Read the model definition and answer for the solid it produces. Units are mm, in the model's axes. Face numbers are marked on the shaded views. A direction names the side the tool comes from. Coordinates: 2 decimals unless noted, no trailing zeros. Order: outer loops, then holes, each group sorted by start corner. A loop starts at its lowest first (then second) coordinate and runs counter-clockwise, first axis right, second up. Notation, with made-up numbers: M 16.25,31 L 67.25,31 A33 cw 67.25,65 Z; hole C -28,31.25 d10. An arc over 180 degrees is marked long. Put each result on its own line as item: value.
from build123d import *

# Parameters (mm, degrees)
SKETCH_1_R          = 3
EXTRUDE_1_DEPTH     = 17
SKETCH_2_R          = 1.5
EXTRUDE_2_DEPTH     = 5
CHAMFER_1_SIZE      = 0.5
SKETCH_3_R          = 1.5
SKETCH_3_R_2        = 1.25
CUT_EXTRUDE_3_DEPTH = 1.5
SKETCH_4_W          = 2
SKETCH_4_H          = 2
CUT_EXTRUDE_4_DEPTH = 10
CHAMFER_2_SIZE      = 0.5


with BuildPart() as part:
    # 草图1 → 拉伸1 (new body)
    with BuildSketch(Plane.XY):
        Circle(SKETCH_1_R)
    extrude(amount=EXTRUDE_1_DEPTH)

    # 草图2 → 拉伸2 (add)
    with BuildSketch(Plane.XY.offset(17)):
        Circle(SKETCH_2_R)
    extrude(amount=EXTRUDE_2_DEPTH)

    # 倒角1
    chamfer_1_edges = [part.edges().sort_by_distance(p)[0] for p in [
        (-1.5, 0, 22),
    ]]
    chamfer(chamfer_1_edges, length=CHAMFER_1_SIZE)

    # 草图3 → 拉伸3 (cut)
    with BuildSketch(Plane.XY.offset(17)):
        Circle(SKETCH_3_R)
        Circle(SKETCH_3_R_2, mode=Mode.SUBTRACT)
    extrude(amount=CUT_EXTRUDE_3_DEPTH, mode=Mode.SUBTRACT)

    # 草图4 → 拉伸4 (cut, symmetric)
    with BuildSketch(Plane(origin=(0, 0, 0), x_dir=(0, 0, -1), z_dir=(1, 0, 0))):
        with Locations((-1, 0)):
            Rectangle(SKETCH_4_W, SKETCH_4_H)
    extrude(amount=CUT_EXTRUDE_4_DEPTH, both=True, mode=Mode.SUBTRACT)

    # 倒角2
    chamfer_2_edges = [part.edges().sort_by_distance(p)[0] for p in [
        (0, 3, 0),
        (0, -3, 0),
        (-3, 0, 17),
    ]]
    chamfer(chamfer_2_edges, length=CHAMFER_2_SIZE)


solid = part.part
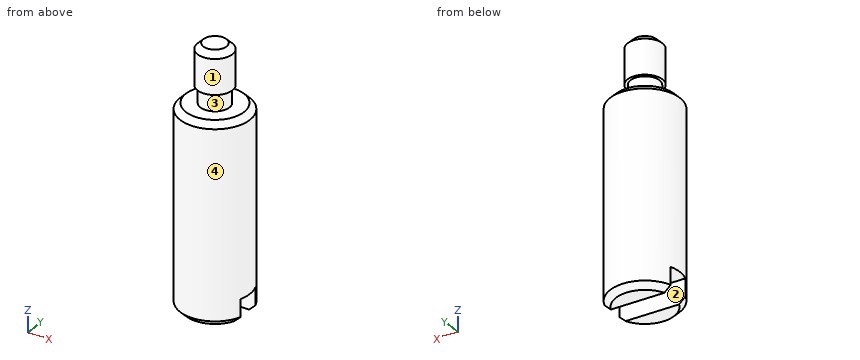
Q1. Find section D-D on z = 19. Write down the section's boundary in (x, y), plus the area to 3 significant figures.
Answers below:
outline: C 0,0 d3
area: 7.07 mm^2
Q2. Given pin 1 (1 mm diameter, centred on y = 1.5, z = 17, fed in from +X); pin 2 (2 mm diameter, centred on x = -2, z = 16.5, fed in from +Y); pin 3 (0.9 mm diameter, centred on x = -0.5, y = -0.5, fed in from -Z), each flat-ended and moving along its own axis, determine where each tip first touches the part or whether it passes through.
Answers below:
pin 1: stops at x = 2.66
pin 2: stops at y = 2.83
pin 3: stops at z = 2
Q3. For a pull along Z with two mould halves and no side action, classify the marked faces 3 and 4 as +Z half, -Z half, draft (parallel to the pull), parting line (faces both ways), or undercut.
Answers below:
face 3: undercut
face 4: draft
Q4. A tool of negligible diameter and unlimited length cuts with its end or side. For the marked faces 1 and 2, from which of +Z, -Z, +X, -X, +Y, -Y can it reach the whole face along a straight path? Write none if from no direction.
Answers below:
face 1: +Z
face 2: -Z, +X, -X
Q5. Consider line 1 along Y through (x, z) = (-2.1, 1.75); line 2 along Z through (x, y) = (0.55, 0.6); line 3 along Z through (x, y) = (0.95, 2.2). Determine where each line is inside the solid, lowest interval first.
Answers below:
line 1: y = -2.14 to -1, 1 to 2.14
line 2: z = 2 to 22
line 3: z = 0 to 17
Q6. Find section C-C on z = 13.75. Write down the section's boundary in (x, y).
Answers below:
outline: C 0,0 d6
Q7. Find section B-B on y = 0. Write down the section's boundary in (x, z), plus the area to 3 significant figures.
Answers below:
outline: M -3,2 L 3,2 L 3,16.5 L 2.5,17 L 1.25,17 L 1.25,18.5 L 1.5,18.5 L 1.5,21.5 L 1,22 L -1,22 L -1.5,21.5 L -1.5,18.5 L -1.25,18.5 L -1.25,17 L -2.5,17 L -3,16.5 Z
area: 104 mm^2
Q8. Find section A-A on x = 0. Write down the section's boundary in (y, z), plus the area to 4 significant figures.
Answers below:
outline: M -3,0.5 L -2.5,0 L -1,0 L -1,2 L 1,2 L 1,0 L 2.5,0 L 3,0.5 L 3,16.5 L 2.5,17 L 1.25,17 L 1.25,18.5 L 1.5,18.5 L 1.5,21.5 L 1,22 L -1,22 L -1.5,21.5 L -1.5,18.5 L -1.25,18.5 L -1.25,17 L -2.5,17 L -3,16.5 Z
area: 111.5 mm^2
